Design review of the part built by this model. Coordinates are the model's own, in mm. Give positions to 0.01 mm unless a question says otherwise; leave off trailing zeros. Loops run counter-clockwise (first coordinate to the right, second up) from the corner with the lowest first, then second, coordinate; pieces in that order, holes last. Notation, with made-up numbers: (50, -35) - (91, -35) arc R28 ccw to (91, -13) - close; hole circle Ø7 at (36.25, 85). An arc over 180 degrees is marked (long way). Put each result on its own line as item: value. Start each with the question number.
```python
from build123d import *

# Parameters (mm, degrees)
SKETCH1_W           = 200
SKETCH1_H           = 300
BOSS_EXTRUDE1_DEPTH = 16
SKETCH2_R           = 5
CUT_EXTRUDE3_DEPTH  = 317.632278835
LPATTERN1_COUNT     = 13
LPATTERN1_PITCH     = 22.5


with BuildPart() as part:
    # Sketch1 → Boss-Extrude1 (new body)
    with BuildSketch(Plane.XY):
        with Locations((0, 150)):
            Rectangle(SKETCH1_W, SKETCH1_H)
    extrude(amount=BOSS_EXTRUDE1_DEPTH)

    # Sketch2 → Cut-Extrude3 (cut, symmetric)
    with BuildSketch(Plane.XY.offset(16)):
        with Locations((90, 12.5)):
            Circle(SKETCH2_R)
    cut_extrude3 = extrude(amount=CUT_EXTRUDE3_DEPTH, both=True, mode=Mode.SUBTRACT)

    # LPattern1: Cut-Extrude3 ×13
    with Locations(*[(0, i * LPATTERN1_PITCH, 0) for i in range(1, LPATTERN1_COUNT)]):
        add(cut_extrude3, mode=Mode.SUBTRACT)


solid = part.part
```
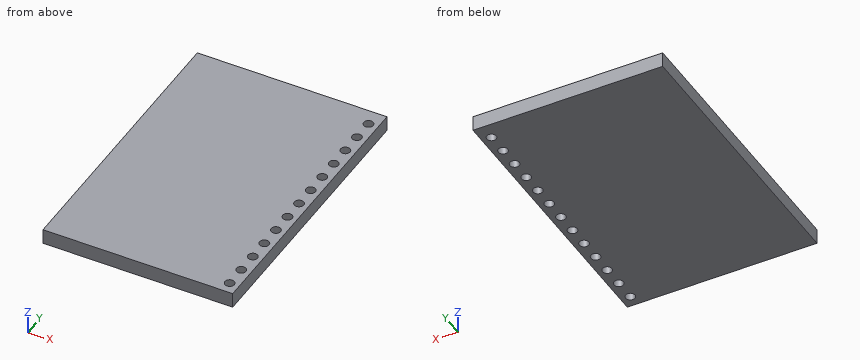
Item 1: Consider section B-B (z = 8.75). Count the separate pieces of the cut face and the enclosed holes in it, plus the area to 3 significant figures.
Item 2: For L1, parallel to X at y = 260, z = 12; L2, parallel to X at y = 83, z = 15.75, list the stretches that pass through material, from the lowest coordinate up. Write a range as from..to.
Item 3: Consider section A-A (y = 125). State the section outline as (x, z) points, plus the area to 3 significant figures.
Item 4: For P1, Ø8, axis at x = 90, y = 237.5, coming from the +Z side; P2, Ø16, axis at x = 90, y = 170, coming from the +Z side, all flat-tipped, find the tip position at first contact; note any pin that passes through.
Geometry says:
1. separate pieces: 1
1. enclosed holes: 13
1. area: 59,000 mm2
2. L1: x = -100..85, 95..100
2. L2: x = -100..86, 94..100
3. outline: (-100, 0) - (85, 0) - (85, 16) - (-100, 16) - close; (95, 0) - (100, 0) - (100, 16) - (95, 16) - close
3. area: 3,040 mm2
4. P1: passes through
4. P2: stops at z = 16
